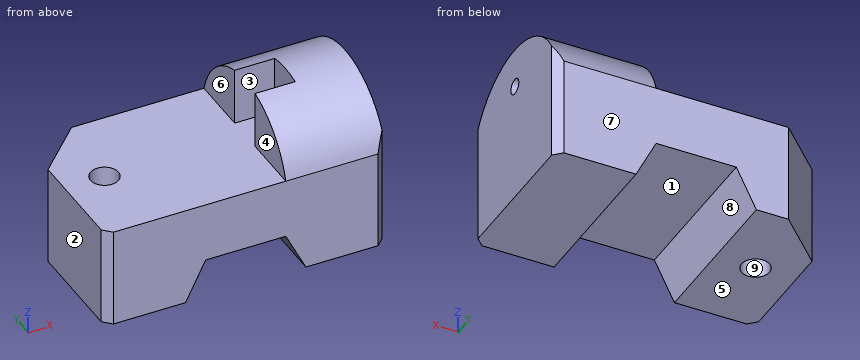
```python
from build123d import *

# Parameters (mm, degrees)
SKETCH1_R           = 3.5
BOSS_EXTRUDE1_DEPTH = 12.5
CUT_EXTRUDE1_DEPTH  = 55.60082417
BOSS_EXTRUDE3_DEPTH = 25
CUT_EXTRUDE2_DEPTH  = 57.789083458
SKETCH8_W           = 10
SKETCH8_H           = 10
CUT_EXTRUDE3_DEPTH  = 48.434164903
SKETCH9_R           = 1.934793031
CUT_EXTRUDE4_DEPTH  = 65.662585782


with BuildPart() as part:
    # Sketch1 → Boss-Extrude1 (new, symmetric)
    with BuildSketch(Plane.XY):
        Polygon((-23, 20), (-35, 8), (-35, -18), (-33, -20), (33, -20), (35, -18), (35, 18), (33, 20), align=None)
        with Locations((-25, 0)):
            Circle(SKETCH1_R, mode=Mode.SUBTRACT)
    extrude(amount=BOSS_EXTRUDE1_DEPTH, both=True)

    # Sketch2 → Cut-Extrude1 (cut, through all)
    with BuildSketch(Plane.XZ.offset(20)):
        Polygon((-10, -2.5), (10, -2.5), (15, -12.5), (-15, -12.5), align=None)
    extrude(amount=-CUT_EXTRUDE1_DEPTH, mode=Mode.SUBTRACT)

    # Sketch5 → Boss-Extrude3 (add)
    with BuildSketch(Plane(origin=(35, 0, 0), x_dir=(0, 0, -1), z_dir=(1, 0, 0))):
        with BuildLine():
            Line((-12.5, 20), (-12.5, -20))
            ThreePointArc((-12.5, -20), (-27.5, 0), (-12.5, 20))
        make_face()
    extrude(amount=-BOSS_EXTRUDE3_DEPTH)

    # Sketch6 → Cut-Extrude2 (cut, through all)
    with BuildSketch(Plane(origin=(0, 0, -12.5), x_dir=(-1, 0, 0), z_dir=(0, 0, -1))):
        Polygon((-35, 20), (-35, 18), (-33, 20), align=None)
        Polygon((-35, -20), (-33, -20), (-35, -18), align=None)
    extrude(amount=-CUT_EXTRUDE2_DEPTH, mode=Mode.SUBTRACT)

    # Sketch8 → Cut-Extrude3 (cut, through all)
    with BuildSketch(Plane.XY.offset(12.5)):
        with Locations((15, 0)):
            Rectangle(SKETCH8_W, SKETCH8_H)
    extrude(amount=CUT_EXTRUDE3_DEPTH, mode=Mode.SUBTRACT)

    # Sketch9 → Cut-Extrude4 (cut, through all)
    with BuildSketch(Plane.ZY.offset(-20)):
        with Locations((17.540032759, 0)):
            Circle(SKETCH9_R)
    extrude(amount=-CUT_EXTRUDE4_DEPTH, mode=Mode.SUBTRACT)


solid = part.part
```
For this review, take the finished solid that the model builds, in its own axes (mm). Face numbers are marked on the shaded views. A direction names the side the tool comes from. Round coordinates to 2 decimals unless told otherwise and drop trailing zeros. Write each loop counter-clockwise with the first axis right and the second up, starting at its lowest first coordinate (ties: lowest second). Pieces come first, ordered by that corner, then holes. Notation, with made-up numbers: M 70,11 L 114,11 A33 ccw 114,40 Z; hole C 27.5,69.5 d8. An arc over 180 degrees is marked long. One line per item, written item: value. Start each with the question number.
(1) The part is to be moulded in two halves that separate along X. For the marked faces 6, 7, 8 and 9, say which applies: released by +X, released by -X, zero draft, split by the parting line, or undercut.
(2) We need section D-D (x = 26). Give the boundary of the cut face in (y, z), and give its area (3 significant figures).
(3) Wall thickness on line 1 (Y direction, x = -25, z = 4.5); line 2 (X direction, y = -6, z = -3); line 3 (Z direction, x = -16, y = -1.5): over which ranges is each line inside the solid? List them lowest first.
(4) We need section C-C (y = 0). Give the boundary of the cut face in (x, z).
(5) We need section B-B (x = -25). Give the boundary of the cut face in (y, z).
(6) Machinability: for the marked faces 1, 2, 3, 4 and 5, which of the approach directions +Z, -Z, +X, -X, +Y, -Y give a long, thin tool a straight path to every point of the face, cutting with its end or side? Answer none if there is none.
(7) We need section A-A (z = -10). Give the boundary of the cut face in (x, y).
(8) Insertion check: pin 1 (20 mm diameter, centred on x = 3, y = 10, fed in from +Z); pin 2 (4.5 mm diameter, centred on y = 15, z = 19, fed in from -X); pin 3 (2 mm diameter, centred on x = -1.5, y = -4.5, fed in from +Z); pin 4 (2.5 mm diameter, centred on y = 0, z = 17.54, fed in from +X). Each pin has a flat end and moves straight along its axis. Give the tip position at first contact, or say it passes through.
Result:
1. face 6: released by -X
1. face 7: zero draft
1. face 8: undercut
1. face 9: undercut
2. outline: M -20,-12.5 L 20,-12.5 L 20,12.5 A20.83 ccw -20,12.5 Z; hole C 0,17.54 d3.87
2. area: 1,430 mm²
3. line 1: -20 to -3.5, 3.5 to 18
3. line 2: -35 to -10.25, 10.25 to 35
3. line 3: -12.5 to 12.5
4. outline: M -35,-12.5 L -28.5,-12.5 L -28.5,12.5 L -35,12.5 Z; M -21.5,-12.5 L -15,-12.5 L -10,-2.5 L 10,-2.5 L 15,-12.5 L 35,-12.5 L 35,15.61 L 20,15.61 L 20,12.5 L -21.5,12.5 Z; M 20,19.47 L 35,19.47 L 35,27.5 L 20,27.5 Z
5. outline: M -20,-12.5 L -3.5,-12.5 L -3.5,12.5 L -20,12.5 Z; M 3.5,-12.5 L 18,-12.5 L 18,12.5 L 3.5,12.5 Z
6. face 1: -Z, +Y, -Y
6. face 2: +Z, -Z, -X, +Y, -Y
6. face 3: +Z, -X
6. face 4: +Z, -X, +Y, -Y
6. face 5: -Z, +X, -X, +Y, -Y
7. outline: M -35,-18 L -33,-20 L -13.75,-20 L -13.75,20 L -23,20 L -35,8 Z; M 13.75,-20 L 33,-20 L 35,-18 L 35,18 L 33,20 L 13.75,20 Z; hole C -25,0 d7
8. pin 1: z = 26.89
8. pin 2: x = 10
8. pin 3: z = 12.5
8. pin 4: through
